Can you work these out from the model? Positions are in its coordinate system, mm. A direction names the side the tool comes from. Coordinates: 2 decimals unless noted, no trailing zeros. Order: outer loops, then holes, each group sorted by start corner. A loop starts at its lowest first (then second) coordinate and runs counter-clockwise, first axis right, second up.
```python
from build123d import *

# Parameters (mm, degrees)
SKETCH_1_R          = 28.5
EXTRUDE_1_DEPTH     = 53.3
SKETCH_2_R          = 17.5
CUT_EXTRUDE_2_DEPTH = 4
SKETCH_2_5_R        = 1.5
CUT_EXTRUDE_3_DEPTH = 5
SKETCH_4_R          = 1.5
CUT_EXTRUDE_4_DEPTH = 4
SKETCH_9_W          = 14
SKETCH_9_H          = 5
CUT_EXTRUDE_6_DEPTH = 3
SKETCH_10_W         = 8
SKETCH_10_H         = 8
CUT_EXTRUDE_7_DEPTH = 3


with BuildPart() as part:
    # 草图1 → 凸台-拉伸1 (new body)
    with BuildSketch(Plane.XY):
        Circle(SKETCH_1_R)
    extrude(amount=EXTRUDE_1_DEPTH)

    # 草图2 → 切除-拉伸2 (cut)
    with BuildSketch(Plane.XY.offset(53.3)):
        Circle(SKETCH_2_R)
    extrude(amount=-CUT_EXTRUDE_2_DEPTH, mode=Mode.SUBTRACT)

    # 草图2<5> → 切除-拉伸3 (cut)
    with BuildSketch(Plane.XY.offset(53.3)):
        with Locations((0, 25)):
            Circle(SKETCH_2_5_R)
        with Locations((21.650635095, 12.5)):
            Circle(SKETCH_2_5_R)
        with Locations((21.650635095, -12.5)):
            Circle(SKETCH_2_5_R)
        with Locations((0, -25)):
            Circle(SKETCH_2_5_R)
        with Locations((-21.650635095, -12.5)):
            Circle(SKETCH_2_5_R)
        with Locations((-21.650635095, 12.5)):
            Circle(SKETCH_2_5_R)
    extrude(amount=-CUT_EXTRUDE_3_DEPTH, mode=Mode.SUBTRACT)

    # 草图4 → 切除-拉伸4 (cut)
    with BuildSketch(Plane(origin=(0, 0, 0), x_dir=(-1, 0, 0), z_dir=(0, 0, -1))):
        with Locations((13.435028843, 13.435028843)):
            Circle(SKETCH_4_R)
        with Locations((-13.435028843, 13.435028843)):
            Circle(SKETCH_4_R)
        with Locations((13.435028843, -13.435028843)):
            Circle(SKETCH_4_R)
        with Locations((-13.435028843, -13.435028843)):
            Circle(SKETCH_4_R)
    extrude(amount=-CUT_EXTRUDE_4_DEPTH, mode=Mode.SUBTRACT)

    # 草图9 → 切除-拉伸6 (cut)
    with BuildSketch(Plane(origin=(0, 28.5, 0), x_dir=(1, 0, 0), z_dir=(0, 1, 0))):
        with Locations((0, -3.5)):
            Rectangle(SKETCH_9_W, SKETCH_9_H)
    cut_extrude_6 = extrude(amount=-CUT_EXTRUDE_6_DEPTH, mode=Mode.SUBTRACT)

    # 镜向1: 切除-拉伸6 across plane
    add(cut_extrude_6.mirror(Plane.ZX), mode=Mode.SUBTRACT)

    # 草图10 → 切除-拉伸7 (cut)
    with BuildSketch(Plane(origin=(-28.5, 0, 0), x_dir=(0, 0, -1), z_dir=(1, 0, 0))):
        with Locations((-5, 0)):
            Rectangle(SKETCH_10_W, SKETCH_10_H)
    extrude(amount=CUT_EXTRUDE_7_DEPTH, mode=Mode.SUBTRACT)


solid = part.part
```
1. Imagine slicing it at A-A on z = 3. Please give me the cut outline in (x, y).
Completed:
outline: (-28.22, -4) arc R28.5 ccw to (-7, -27.63) - (-7, -25.5) - (7, -25.5) - (7, -27.63) arc R28.5 ccw to (7, 27.63) - (7, 25.5) - (-7, 25.5) - (-7, 27.63) arc R28.5 ccw to (-28.22, 4) - (-25.5, 4) - (-25.5, -4) - close; hole circle Ø3 at (-13.44, -13.44); hole circle Ø3 at (-13.44, 13.44); hole circle Ø3 at (13.44, -13.44); hole circle Ø3 at (13.44, 13.44)
2. Imagine slicing it at D-D on x = -22. Please give me the cut outline in (y, z).
Completed:
outline: (-18.12, 0) - (18.12, 0) - (18.12, 53.3) - (13.96, 53.3) - (13.96, 48.3) - (11.04, 48.3) - (11.04, 53.3) - (-11.04, 53.3) - (-11.04, 48.3) - (-13.96, 48.3) - (-13.96, 53.3) - (-18.12, 53.3) - close
3. Imagine slicing it at B-B on x = 0. Please give me the cut outline in (y, z), then the cut area to 3 significant figures.
Completed:
outline: (-28.5, 0) - (28.5, 0) - (28.5, 1) - (25.5, 1) - (25.5, 6) - (28.5, 6) - (28.5, 53.3) - (26.5, 53.3) - (26.5, 48.3) - (23.5, 48.3) - (23.5, 53.3) - (17.5, 53.3) - (17.5, 49.3) - (-17.5, 49.3) - (-17.5, 53.3) - (-23.5, 53.3) - (-23.5, 48.3) - (-26.5, 48.3) - (-26.5, 53.3) - (-28.5, 53.3) - (-28.5, 6) - (-25.5, 6) - (-25.5, 1) - (-28.5, 1) - close
area: 2,840 mm2
4. I'm going to push flat-ended pins straight in: pin 1 (1 mm diameter, centred on x = 11.5, z = 14, fed in from -Y); pin 2 (0.6 mm diameter, centred on y = -26.5, z = 2.5, fed in from +X); pin 3 (5.5 mm diameter, centred on x = 1, z = 4.5, fed in from +Y); pin 4 (3.5 mm diameter, centred on x = -21, y = -13, fed in from +Z). Where does each tip first touch, or does it pass through?
Completed:
pin 1: stops at y = -26.29
pin 2: stops at x = 11.22
pin 3: stops at y = 28.5
pin 4: stops at z = 53.3
5. Thinking about a two-plate mould opening in Y: for faces 5 (the flat face through (0, 25.5, 3)), 6 (the flat face through (7, -27, 4)), 7 (the cylindrical face through (23.08, 12.95, 50.83)), 8 (the cylindrical face through (27.184, 8.561, 26.277)), which applies, pulls with the +Y half, pulls with the -Y half, needs draft (parallel to the pull), parting line crosses it, or undercut?
Completed:
face 5: pulls with the +Y half
face 6: needs draft
face 7: undercut
face 8: parting line crosses it
6. Imagine slicing it at C-C on y = 6.5. Please give me the cut outline in (x, z), then the cut area to 3 significant figures.
Completed:
outline: (-27.75, 0) - (27.75, 0) - (27.75, 53.3) - (16.25, 53.3) - (16.25, 49.3) - (-16.25, 49.3) - (-16.25, 53.3) - (-27.75, 53.3) - close
area: 2,830 mm2
7. Please list where these lines run through material, in increasing order: probe 1 along Y at (x, z) = (0, 51.9); probe 2 along Z at (x, y) = (-7.5, 9.5); probe 3 along X at (y, z) = (-7, 16).
Completed:
probe 1: y = -28.5 to -26.5, -23.5 to -17.5, 17.5 to 23.5, 26.5 to 28.5
probe 2: z = 0 to 49.3
probe 3: x = -27.63 to 27.63
8. On a 3-axis mill with a long thin cutter (end or side, diameter ignored), from which of +Z, -Z, +X, -X, +Y, -Y can I reach the whole of each face in a straight line? I mean faces 1 (the flat face through (22, -12, 48.3)), 2 (the cylindrical face through (-14.82, -14.01, 1.97)), 3 (the flat face through (-25.5, 0, 5)), 4 (the flat face through (0, -25.5, 3)). Say none if no direction works.
Completed:
face 1: +Z
face 2: -Z
face 3: -X
face 4: -Y
